```python
from build123d import *

# Parameters (mm, degrees)
SKETCH1_W           = 164.1
SKETCH1_H           = 174.745
SKETCH1_R           = 2.5527
BOSS_EXTRUDE1_DEPTH = 1.5875
FILLET1_R           = 1


with BuildPart() as part:
    # Sketch1 → Boss-Extrude1 (new body)
    with BuildSketch(Plane.XY):
        with Locations((82.55, -87.3725)):
            Rectangle(SKETCH1_W, SKETCH1_H)
        with Locations((82.55, -87.3725)):
            Circle(SKETCH1_R, mode=Mode.SUBTRACT)
        with BuildLine():
            Line((82.55, -5.4375), (80.434372699, -5.4375))
            ThreePointArc((80.434372699, -5.4375), (75.6625, -3.85), (80.434372699, -2.2625))
            Line((80.434372699, -2.2625), (82.55, -2.2625))
            ThreePointArc((82.55, -2.2625), (84.1375, -3.85), (82.55, -5.4375))
        make_face(mode=Mode.SUBTRACT)
        with BuildLine():
            Line((16.934372699, -168.395), (19.05, -168.395))
            ThreePointArc((19.05, -168.395), (20.6375, -169.9825), (19.05, -171.57))
            Line((19.05, -171.57), (16.934372699, -171.57))
            ThreePointArc((16.934372699, -171.57), (12.1625, -169.9825), (16.934372699, -168.395))
        make_face(mode=Mode.SUBTRACT)
        with BuildLine():
            Line((7.409372699, -151.9325), (9.525, -151.9325))
            ThreePointArc((9.525, -151.9325), (11.1125, -153.52), (9.525, -155.1075))
            Line((9.525, -155.1075), (7.409372699, -155.1075))
            ThreePointArc((7.409372699, -155.1075), (2.6375, -153.52), (7.409372699, -151.9325))
        make_face(mode=Mode.SUBTRACT)
        with BuildLine():
            Line((42.334372699, -168.395), (44.45, -168.395))
            ThreePointArc((44.45, -168.395), (46.0375, -169.9825), (44.45, -171.57))
            Line((44.45, -171.57), (42.334372699, -171.57))
            ThreePointArc((42.334372699, -171.57), (37.5625, -169.9825), (42.334372699, -168.395))
        make_face(mode=Mode.SUBTRACT)
        with BuildLine():
            Line((67.734372699, -168.395), (69.85, -168.395))
            ThreePointArc((69.85, -168.395), (71.4375, -169.9825), (69.85, -171.57))
            Line((69.85, -171.57), (67.734372699, -171.57))
            ThreePointArc((67.734372699, -171.57), (62.9625, -169.9825), (67.734372699, -168.395))
        make_face(mode=Mode.SUBTRACT)
        with BuildLine():
            Line((7.409372699, -126.5325), (9.525, -126.5325))
            ThreePointArc((9.525, -126.5325), (11.1125, -128.12), (9.525, -129.7075))
            Line((9.525, -129.7075), (7.409372699, -129.7075))
            ThreePointArc((7.409372699, -129.7075), (2.6375, -128.12), (7.409372699, -126.5325))
        make_face(mode=Mode.SUBTRACT)
        with BuildLine():
            Line((7.409372699, -101.1325), (9.525, -101.1325))
            ThreePointArc((9.525, -101.1325), (11.1125, -102.72), (9.525, -104.3075))
            Line((9.525, -104.3075), (7.409372699, -104.3075))
            ThreePointArc((7.409372699, -104.3075), (2.6375, -102.72), (7.409372699, -101.1325))
        make_face(mode=Mode.SUBTRACT)
        with BuildLine():
            Line((7.409372699, -75.7325), (9.525, -75.7325))
            ThreePointArc((9.525, -75.7325), (11.1125, -77.32), (9.525, -78.9075))
            Line((9.525, -78.9075), (7.409372699, -78.9075))
            ThreePointArc((7.409372699, -78.9075), (2.6375, -77.32), (7.409372699, -75.7325))
        make_face(mode=Mode.SUBTRACT)
        with BuildLine():
            Line((7.409372699, -50.3325), (9.525, -50.3325))
            ThreePointArc((9.525, -50.3325), (11.1125, -51.92), (9.525, -53.5075))
            Line((9.525, -53.5075), (7.409372699, -53.5075))
            ThreePointArc((7.409372699, -53.5075), (2.6375, -51.92), (7.409372699, -50.3325))
        make_face(mode=Mode.SUBTRACT)
        with BuildLine():
            Line((7.409372699, -24.9325), (9.525, -24.9325))
            ThreePointArc((9.525, -24.9325), (11.1125, -26.52), (9.525, -28.1075))
            Line((9.525, -28.1075), (7.409372699, -28.1075))
            ThreePointArc((7.409372699, -28.1075), (2.6375, -26.52), (7.409372699, -24.9325))
        make_face(mode=Mode.SUBTRACT)
        with BuildLine():
            Line((7.409372699, -8.1), (9.525, -8.1))
            ThreePointArc((9.525, -8.1), (11.1125, -9.6875), (9.525, -11.275))
            Line((9.525, -11.275), (7.409372699, -11.275))
            ThreePointArc((7.409372699, -11.275), (2.6375, -9.6875), (7.409372699, -8.1))
        make_face(mode=Mode.SUBTRACT)
        with BuildLine():
            Line((29.634372699, -2.2625), (31.75, -2.2625))
            ThreePointArc((31.75, -2.2625), (33.3375, -3.85), (31.75, -5.4375))
            Line((31.75, -5.4375), (29.634372699, -5.4375))
            ThreePointArc((29.634372699, -5.4375), (24.8625, -3.85), (29.634372699, -2.2625))
        make_face(mode=Mode.SUBTRACT)
        with BuildLine():
            Line((55.034372699, -2.2625), (57.15, -2.2625))
            ThreePointArc((57.15, -2.2625), (58.7375, -3.85), (57.15, -5.4375))
            Line((57.15, -5.4375), (55.034372699, -5.4375))
            ThreePointArc((55.034372699, -5.4375), (50.2625, -3.85), (55.034372699, -2.2625))
        make_face(mode=Mode.SUBTRACT)
        with BuildLine():
            ThreePointArc((161.925, -8.1), (163.5125, -9.6875), (161.925, -11.275))
            Line((161.925, -11.275), (159.809372699, -11.275))
            ThreePointArc((159.809372699, -11.275), (155.0375, -9.6875), (159.809372699, -8.1))
            Line((159.809372699, -8.1), (161.925, -8.1))
        make_face(mode=Mode.SUBTRACT)
        with BuildLine():
            Line((93.134372699, -168.395), (95.25, -168.395))
            ThreePointArc((95.25, -168.395), (96.8375, -169.9825), (95.25, -171.57))
            Line((95.25, -171.57), (93.134372699, -171.57))
            ThreePointArc((93.134372699, -171.57), (88.3625, -169.9825), (93.134372699, -168.395))
        make_face(mode=Mode.SUBTRACT)
        with BuildLine():
            Line((118.534372699, -168.395), (120.65, -168.395))
            ThreePointArc((120.65, -168.395), (122.2375, -169.9825), (120.65, -171.57))
            Line((120.65, -171.57), (118.534372699, -171.57))
            ThreePointArc((118.534372699, -171.57), (113.7625, -169.9825), (118.534372699, -168.395))
        make_face(mode=Mode.SUBTRACT)
        with BuildLine():
            Line((143.934372699, -168.395), (146.05, -168.395))
            ThreePointArc((146.05, -168.395), (147.6375, -169.9825), (146.05, -171.57))
            Line((146.05, -171.57), (143.934372699, -171.57))
            ThreePointArc((143.934372699, -171.57), (139.1625, -169.9825), (143.934372699, -168.395))
        make_face(mode=Mode.SUBTRACT)
        with BuildLine():
            Line((159.809372699, -151.9325), (161.925, -151.9325))
            ThreePointArc((161.925, -151.9325), (163.5125, -153.52), (161.925, -155.1075))
            Line((161.925, -155.1075), (159.809372699, -155.1075))
            ThreePointArc((159.809372699, -155.1075), (155.0375, -153.52), (159.809372699, -151.9325))
        make_face(mode=Mode.SUBTRACT)
        with BuildLine():
            Line((159.809372699, -126.5325), (161.925, -126.5325))
            ThreePointArc((161.925, -126.5325), (163.5125, -128.12), (161.925, -129.7075))
            Line((161.925, -129.7075), (159.809372699, -129.7075))
            ThreePointArc((159.809372699, -129.7075), (155.0375, -128.12), (159.809372699, -126.5325))
        make_face(mode=Mode.SUBTRACT)
        with BuildLine():
            Line((159.809372699, -101.1325), (161.925, -101.1325))
            ThreePointArc((161.925, -101.1325), (163.5125, -102.72), (161.925, -104.3075))
            Line((161.925, -104.3075), (159.809372699, -104.3075))
            ThreePointArc((159.809372699, -104.3075), (155.0375, -102.72), (159.809372699, -101.1325))
        make_face(mode=Mode.SUBTRACT)
        with BuildLine():
            Line((159.809372699, -75.7325), (161.925, -75.7325))
            ThreePointArc((161.925, -75.7325), (163.5125, -77.32), (161.925, -78.9075))
            Line((161.925, -78.9075), (159.809372699, -78.9075))
            ThreePointArc((159.809372699, -78.9075), (155.0375, -77.32), (159.809372699, -75.7325))
        make_face(mode=Mode.SUBTRACT)
        with BuildLine():
            Line((159.809372699, -50.3325), (161.925, -50.3325))
            ThreePointArc((161.925, -50.3325), (163.5125, -51.92), (161.925, -53.5075))
            Line((161.925, -53.5075), (159.809372699, -53.5075))
            ThreePointArc((159.809372699, -53.5075), (155.0375, -51.92), (159.809372699, -50.3325))
        make_face(mode=Mode.SUBTRACT)
        with BuildLine():
            Line((105.834372699, -2.2625), (107.95, -2.2625))
            ThreePointArc((107.95, -2.2625), (109.5375, -3.85), (107.95, -5.4375))
            Line((107.95, -5.4375), (105.834372699, -5.4375))
            ThreePointArc((105.834372699, -5.4375), (101.0625, -3.85), (105.834372699, -2.2625))
        make_face(mode=Mode.SUBTRACT)
        with BuildLine():
            Line((159.809372699, -24.9325), (161.925, -24.9325))
            ThreePointArc((161.925, -24.9325), (163.5125, -26.52), (161.925, -28.1075))
            Line((161.925, -28.1075), (159.809372699, -28.1075))
            ThreePointArc((159.809372699, -28.1075), (155.0375, -26.52), (159.809372699, -24.9325))
        make_face(mode=Mode.SUBTRACT)
        with BuildLine():
            Line((131.234372699, -2.2625), (133.35, -2.2625))
            ThreePointArc((133.35, -2.2625), (134.9375, -3.85), (133.35, -5.4375))
            Line((133.35, -5.4375), (131.234372699, -5.4375))
            ThreePointArc((131.234372699, -5.4375), (126.4625, -3.85), (131.234372699, -2.2625))
        make_face(mode=Mode.SUBTRACT)
    extrude(amount=BOSS_EXTRUDE1_DEPTH)

    # Fillet1
    fillet1_edges = [part.edges().sort_by_distance(p)[0] for p in [
        (0.5, -174.745, 0.79375),
        (0.5, 0, 0.79375),
        (164.6, 0, 0.79375),
        (164.6, -174.745, 0.79375),
    ]]
    fillet(fillet1_edges, radius=FILLET1_R)


solid = part.part
```
Here's how the part is built. I have some questions about the finished solid (model axes, mm). Coordinates: 2 decimals unless noted, no trailing zeros. Order: outer loops, then holes, each group sorted by start corner. A loop starts at its lowest first (then second) coordinate and runs counter-clockwise, first axis right, second up.
Item 1: I need wall thicknesses on probe 1 along X at (y, z) = (-77.32, 1.05); probe 2 along X at (y, z) = (-52.5, 1.2); probe 3 along Y at (x, z) = (43.5, 0.85) (3 decimals). Which ranges of each line are inside material? Lowest first, please.
Response values:
probe 1: x = 0.5 to 2.64, 11.11 to 155.04, 163.51 to 164.6
probe 2: x = 0.5 to 2.7, 11 to 155.1, 163.4 to 164.6
probe 3: y = -174.745 to -171.57, -168.395 to 0
Item 2: Thinking about a two-plate mould opening in Y: for faces 1 (the face through (100, -86, 0)), 2 (the face through (139.164, -170.075, 0.783)), which applies, pulls with the +Y half, pulls with the -Y half, needs draft (parallel to the pull), parting line crosses it, or undercut?
Response values:
face 1: needs draft
face 2: undercut
Item 3: If we section it at C-C, the plane z = 0.85: Give the number of separate pieces and of enclosed holes in the cut face, then the cut area to 3 significant figures.
Response values:
separate pieces: 1
enclosed holes: 26
area: 27,900 mm2
Item 4: If we section it at B-B, the plane x = 103: List the corners of the cut face in (y, z) for me (1 decimal), then the cut area to 3 significant figures.
Response values:
outline: (-174.7, 0) - (-6.4, 0) - (-6.4, 1.6) - (-174.7, 1.6) - close; (-1.3, 0) - (0, 0) - (0, 1.6) - (-1.3, 1.6) - close
area: 269 mm2
Item 5: If we section it at A-A, the plane x = 65.5: List the corners of the cut face in (y, z) for me (1 decimal).
Response values:
outline: (-174.7, 0) - (-172.6, 0) - (-172.6, 1.6) - (-174.7, 1.6) - close; (-167.3, 0) - (0, 0) - (0, 1.6) - (-167.3, 1.6) - close
